Design review of the part built by this model. Coordinates are the model's own, in mm. A direction names the side the tool comes from. Give positions to 0.01 mm unless a question says otherwise; leave off trailing zeros. Loops run counter-clockwise (first coordinate to the right, second up) from the corner with the lowest first, then second, coordinate; pieces in that order, holes last. Notation, with made-up numbers: (32, -40) - (73, -40) arc R7 cw to (73, -30) - close; hole circle Ø2 at (64, 17.5). An arc over 180 degrees is marked (long way). Write each question's results on one line, items separated by ' | '.
```python
from build123d import *

# Parameters (mm, degrees)
EXTRUDE_1_DEPTH     = 8
FILLET_2_R          = 3
FILLET_3_R          = 3
FILLET_4_R          = 3
FILLET_5_R          = 3
FILLET_6_R          = 3
FILLET_7_R          = 3
SKETCH_3_R          = 1.5
CUT_EXTRUDE_1_DEPTH = 20
SKETCH_4_R          = 1.5
CUT_EXTRUDE_2_DEPTH = 20


with BuildPart() as part:
    # 草图1 → 凸台-拉伸1 (new body)
    with BuildSketch(Plane(origin=(0, 0, 0), x_dir=(1, 0, 0), z_dir=(0, 1, 0))):
        with BuildLine():
            Line((8.935144768, 1), (13, 1))
            Line((13, 1), (13, 2))
            Line((13, 2), (5.123475383, 2))
            ThreePointArc((5.123475383, 2), (1.206089666, 5.366129678), (-3.774917218, 4))
            Line((-3.774917218, 4), (-11, 4))
            Line((-11, 4), (-11, -4))
            Line((-11, -4), (-3.774917218, -4))
            ThreePointArc((-3.774917218, -4), (1.206089666, -5.366129678), (5.123475383, -2))
            Line((5.123475383, -2), (12.990817457, -2))
            Line((12.990817457, -2), (12.995479361, -1))
            Line((12.995479361, -1), (5.408326913, -1))
            Line((5.408326913, -1), (3.872983346, -1))
            ThreePointArc((3.872983346, -1), (-4, 0), (3.872983346, 1))
            Line((3.872983346, 1), (8.935144768, 1))
        make_face()
    extrude(amount=EXTRUDE_1_DEPTH)

    # 圆角2
    fillet_2_edges = [part.edges().sort_by_distance(p)[0] for p in [
        (-11, 8, 0),
    ]]
    fillet(fillet_2_edges, radius=FILLET_2_R)

    # 圆角3
    fillet_3_edges = [part.edges().sort_by_distance(p)[0] for p in [
        (-11, 0, 0),
    ]]
    fillet(fillet_3_edges, radius=FILLET_3_R)

    # 圆角4
    fillet_4_edges = [part.edges().sort_by_distance(p)[0] for p in [
        (12.993148409, 8, 1.5),
    ]]
    fillet(fillet_4_edges, radius=FILLET_4_R)

    # 圆角5
    fillet_5_edges = [part.edges().sort_by_distance(p)[0] for p in [
        (12.993148409, 0, 1.5),
    ]]
    fillet(fillet_5_edges, radius=FILLET_5_R)

    # 圆角6
    fillet_6_edges = [part.edges().sort_by_distance(p)[0] for p in [
        (13, 8, -1.5),
    ]]
    fillet(fillet_6_edges, radius=FILLET_6_R)

    # 圆角7
    fillet_7_edges = [part.edges().sort_by_distance(p)[0] for p in [
        (13, 0, -1.5),
    ]]
    fillet(fillet_7_edges, radius=FILLET_7_R)

    # 草图3 → 切除-拉伸1 (cut)
    with BuildSketch(Plane.XY.offset(4)):
        with Locations((-8, 4)):
            Circle(SKETCH_3_R)
    extrude(amount=-CUT_EXTRUDE_1_DEPTH, mode=Mode.SUBTRACT)

    # 草图4 → 切除-拉伸2 (cut)
    with BuildSketch(Plane.XY.offset(2)):
        with Locations((9.990817457, 4)):
            Circle(SKETCH_4_R)
    extrude(amount=-CUT_EXTRUDE_2_DEPTH, mode=Mode.SUBTRACT)


solid = part.part
```
Item 1: We need section C-C on x = 6.5. Give the boundary of the cut face in (y, z), then the cut area to 3 significant figures.
Output values:
outline: (0, -2) - (8, -2) - (8, -1) - (0, -1) - close; (0, 1) - (8, 1) - (8, 2) - (0, 2) - close | area: 16.0 mm²
Item 2: We need section B-B on z = 2.25. Give the boundary of the cut face in (x, y), then the cut area to 3 significant figures.
Output values:
outline: (-11, 3) arc R3 ccw to (-8, 0) - (-3.31, 0) - (-3.31, 8) - (-8, 8) arc R3 ccw to (-11, 5) - close; (3.31, 0) - (5.02, 0) - (5.02, 8) - (3.31, 8) - close; hole circle Ø3 at (-8, 4) | area: 64.3 mm²
Item 3: Tool access review of faces 5 (the face through (-6.6, 3.1, 4)), 6 (the face through (8, 4, 2)), 7 (the face through (8, 4, -2)): name each direction out of +Z, -Z, +X, -X, +Y, -Y from which nothing blocks a thin tool from reaching the whole face with its end or side.
Output values:
face 5: +Z, -X, +Y, -Y | face 6: +Z, +X, +Y, -Y | face 7: -Z, +X, +Y, -Y
Item 4: Wall thickness on probe 1 along Z at (x, y) = (0, 1.25); probe 2 along Z at (x, y) = (8.5, 6.5); probe 3 along Y at (x, z) = (-8, 2.25): over which ranges is each line inside the solid? List them lowest first.
Output values:
probe 1: z = -5.5 to -4, 4 to 5.5 | probe 2: z = -2 to -1, 1 to 2 | probe 3: y = 0 to 2.5, 5.5 to 8
Item 5: Clearance check with flat-ended pins moving along their axes: P1, Ø4, axis at x = 11, y = 5.5, coming from the +Z side; P2, Ø2.5, axis at x = 10.5, y = 5.5, coming from the -Z side; P3, Ø2, axis at y = 6, z = -4, coming from the +X side. State where each tip first meets the part, or that it passes through.
Output values:
P1: stops at z = 2 | P2: stops at z = -2 | P3: stops at x = 4.61
Item 6: We need section A-A on y = 4. Give the boundary of the cut face in (x, z), then the cut area to 3 significant figures.
Output values:
outline: (-11, -4) - (-9.5, -4) - (-9.5, 4) - (-11, 4) - close; (-6.5, -4) - (-3.77, -4) arc R5.5 ccw to (5.12, -2) - (8.49, -2) - (8.49, -1) - (3.87, -1) arc R4 cw (long way) to (3.87, 1) - (8.49, 1) - (8.49, 2) - (5.12, 2) arc R5.5 ccw to (-3.77, 4) - (-6.5, 4) - close; (11.49, -2) - (13, -2) - (13, -1) - (11.49, -1) - close; (11.49, 1) - (13, 1) - (12.99, 2) - (11.49, 2) - close | area: 75.4 mm²
Item 7: Draft analysis for pull direction X (two halves, no side actions). For faces 1 (the face through (7, 4, 1)), 2 (the face through (10.797, 5.265, 1.507)), 3 (the face through (-10.14, 7.1, 0.06)), 4 (the face through (13, 4, -1.5)), state which applies: +X half, -X half, draft (parallel to the pull), parting line (faces both ways), or undercut.
Output values:
face 1: draft | face 2: undercut | face 3: -X half | face 4: +X half
Item 8: We need section D-D on z = -1.25. Give the boundary of the cut face in (x, y), then the cut area to 3 significant figures.
Output values:
outline: (-11, 3) arc R3 ccw to (-8, 0) - (-3.8, 0) - (-3.8, 8) - (-8, 8) arc R3 ccw to (-11, 5) - close; (3.8, 0) - (10, 0) arc R3 ccw to (13, 3) - (13, 5) arc R3 ccw to (10, 8) - (3.8, 8) - close; hole circle Ø3 at (-8, 4); hole circle Ø3 at (9.99, 4) | area: 109 mm²
